Could you check a few things on this model? Use its own coordinates, in mm. A direction names the side the tool comes from. Coordinates: 2 decimals unless noted, no trailing zeros. Write each loop counter-clockwise with the first axis right and the second up, starting at its lowest first coordinate (ties: lowest second). Pieces come first, ordered by that corner, then holes. Notation, with made-up numbers: M 0,-14.5 L 7,-14.5 A18 cw 7,-0.5 Z; hole C 83,-14 d6. An arc over 180 degrees is marked long. Answer as CSV lines item,"result". Start each with the question number.
Item 1: If I drill on line 1 along X through (y, z) = (27.5, 0); line 2 along X through (y, z) = (3.15, 42.5); line 3 along Y through (x, z) = (15, 13), over which ranges is the centre line in solid material (lowest first)? Write a range as [from, to].
Item 2: Suppose I cut it at A-A, the plane y = 2.25. Write out the boundary of the cut face in (x, z).
Item 3: Suppose I cut it at C-C, the plane y = 12.5. Write out the boundary of the cut face in (x, z), and give its area (3 significant figures).
Item 4: Suppose I cut it at D-D, the plane y = 17.75. Write out the boundary of the cut face in (x, z).
Item 5: Suppose I cut it at B-B, the plane z = 1. State how many separate pieces and enclosed holes the cut face has, and give its area (3 significant figures).
Item 6: We'd pull the mould along Z, two halves only. Please class faces 4 (the cylindrical face through (-1.844, 2.465, 50.498)), 5 (the flat face through (-32, 5, -21)), 6 (the flat face through (-2, 24, 16)): +Z half, -Z half, draft (parallel to the pull), parting line (faces both ways), or undercut.
Item 7: I'm going to push flat-ended pins straight in: P1, Ø5, axis at x = -8, z = 14, coming from the -Y side; P2, Ø8, axis at y = 4, z = 14, coming from the +X side; P3, Ø1.5, axis at y = 23.5, z = -5.5, coming from the +X side; P4, Ø14, axis at x = -2, z = -16, coming from the +Y side. Where does each tip first touch, or does it pass through?
Item 8: On a 3-axis mill with a long thin cutter (end or side, diameter ignored), from which of +Z, -Z, +X, -X, +Y, -Y can I reach the whole of each face in a straight line? I mean faces 1 (the flat face through (-15, 25, 0)), 2 (the cylindrical face through (-12, 24, 22)), 3 (the flat face through (15, 22, 0)). Say none if no direction works.
```python
from build123d import *

# Parameters (mm, degrees)
SKETCH1_R                = 35
BOSS_EXTRUDE1_DEPTH      = 25
FILLET1_R                = 10
SHELL1_T                 = -3
SKETCH2_R                = 4
BOSS_EXTRUDE2_DEPTH      = 5
CIRPATTERN1_COUNT        = 3
CUT_EXTRUDE2_DEPTH       = 5
LPATTERN2_COUNT          = 7
LPATTERN2_PITCH          = 6
BOSS_EXTRUDE3_DEPTH      = 5
BOSS_EXTRUDE3_DEPTH_BACK = 3
SKETCH8_R                = 12.5
FILLET2_R                = 2
SKETCH9_R                = 7.5
CUT_EXTRUDE3_DEPTH       = 75.49391866


with BuildPart() as part:
    # Sketch1 → Boss-Extrude1 (new body)
    with BuildSketch(Plane(origin=(0, 0, 0), x_dir=(1, 0, 0), z_dir=(0, 1, 0))):
        with Locations(Location((0, 0, 0), (0, 0, 270))):
            Circle(SKETCH1_R)
    extrude(amount=BOSS_EXTRUDE1_DEPTH)

    # Fillet1
    fillet1_edges = [part.edges().sort_by_distance(p)[0] for p in [
        (0, 25, -35),
    ]]
    fillet(fillet1_edges, radius=FILLET1_R)

    # Shell1
    shell1_openings = [part.faces().sort_by_distance(p)[0] for p in [
        (0, 0, 0),
    ]]
    offset(amount=SHELL1_T, openings=shell1_openings, kind=Kind.INTERSECTION)

    # Sketch2 → Boss-Extrude2 (add)
    with BuildSketch(Plane.XZ):
        with BuildLine():
            Line((-10.019580099, 42.5), (-10.019580099, 32))
            Line((-10.019580099, 32), (5.980419901, 32))
            Line((5.980419901, 32), (5.980419901, 42.5))
            ThreePointArc((5.980419901, 42.5), (-2.019580099, 50.5), (-10.019580099, 42.5))
        make_face()
        with Locations(Location((-2.019580099, 42.5, 0), (0, 0, 270))):
            Circle(SKETCH2_R, mode=Mode.SUBTRACT)
    boss_extrude2 = extrude(amount=-BOSS_EXTRUDE2_DEPTH)

    # CirPattern1: Boss-Extrude2 ×3 about axis
    cirpattern1_axis = Axis((0, 0, 0), (0, 1, 0))
    for i in range(1, CIRPATTERN1_COUNT):
        add(boss_extrude2.rotate(cirpattern1_axis, i * 360 / CIRPATTERN1_COUNT))

    # Sketch3 → Cut-Extrude2 (cut)
    with BuildSketch(Plane(origin=(0, 25, 0), x_dir=(1, 0, 0), z_dir=(0, 1, 0))):
        with BuildLine():
            Line((-16, 20), (-16, -20))
            ThreePointArc((-16, -20), (-18, -22), (-20, -20))
            Line((-20, -20), (-20, 20))
            ThreePointArc((-20, 20), (-18, 22), (-16, 20))
        make_face()
    cut_extrude2 = extrude(amount=-CUT_EXTRUDE2_DEPTH, mode=Mode.SUBTRACT)

    # LPattern2: Cut-Extrude2 ×7
    with Locations(*[(i * LPATTERN2_PITCH, 0, 0) for i in range(1, LPATTERN2_COUNT)]):
        add(cut_extrude2, mode=Mode.SUBTRACT)

    # Sketch8 → Boss-Extrude3 (add, two sides: drawn at the far end of the back side and taken through both)
    with BuildSketch(Plane(origin=(0, 25, 0), x_dir=(1, 0, 0), z_dir=(0, 1, 0)).offset(-BOSS_EXTRUDE3_DEPTH_BACK)):
        with Locations(Location((0, 0, 0), (0, 0, 270))):
            Circle(SKETCH8_R)
    extrude(amount=BOSS_EXTRUDE3_DEPTH + BOSS_EXTRUDE3_DEPTH_BACK)

    # Fillet2
    fillet2_edges = [part.edges().sort_by_distance(p)[0] for p in [
        (0, 30, -12.5),
    ]]
    fillet(fillet2_edges, radius=FILLET2_R)

    # Sketch9 → Cut-Extrude3 (cut, through all)
    with BuildSketch(Plane(origin=(0, 30, 0), x_dir=(1, 0, 0), z_dir=(0, 1, 0))):
        with Locations(Location((0, 0, 0), (0, 0, 270))):
            Circle(SKETCH9_R)
    extrude(amount=-CUT_EXTRUDE3_DEPTH, mode=Mode.SUBTRACT)


solid = part.part
```
Ans:
1,line 1,"x = [-12.5, -7.5], [7.5, 12.5]"
1,line 2,"x = [-10.02, -6.02], [1.98, 5.98]"
1,line 3,"y = [22, 25]"
2,outline,"M -39.8,-16.07 A8 ccw -31.8,-29.93 L -24.03,-25.44 A35 ccw 26.87,-22.42 L 33.82,-26.43 A8 ccw 41.82,-12.57 L 34.05,-8.09 A35 ccw 5.98,34.49 L 5.98,42.5 A8 ccw -10.02,42.5 L -10.02,33.54 A35 ccw -32.86,-12.06 Z; hole C -35.8,-23 d8; hole C 0,0 d64; hole C -2.02,42.5 d8; hole C 37.82,-19.5 d8"
3,outline,"C 0,0 d70; hole C 0,0 d64"
3,area,"631 mm^2"
4,outline,"C 0,0 d69.23; hole C 0,0 d62.87"
5,separate pieces,"6"
5,enclosed holes,"0"
5,area,"291 mm^2"
6,face 4,"+Z half"
6,face 5,"draft"
6,face 6,"undercut"
7,P1,"stops at y = 22"
7,P2,"stops at x = 33.54"
7,P3,"stops at x = 30.84"
7,P4,"stops at y = 30"
8,face 1,"+Z, -Z, -X, +Y"
8,face 2,"+Y, -Y"
8,face 3,"-Y"
